Geometry: see drawing. Coordinates: mm, zero at the bounding-box minimum. A direction names the side the tool comes from. Round coordinates to 2 decimals unless told otherwise and drop trailing zeros. Write each loop counter-clockwise with the first axis right and the second up, starting at its lowest first coordinate (ties: lowest second). Pieces come first, ordered by that corner, then holes. Notation, with made-up numbers: (5, 29.5) -> (21, 29.5) arc R24 cw to (21, 47.5) -> close; hole circle Ø3 at (-2.5, -22.5). An arc over 180 degrees is marked (long way). Write item = value, one per line. Start each with the question number.
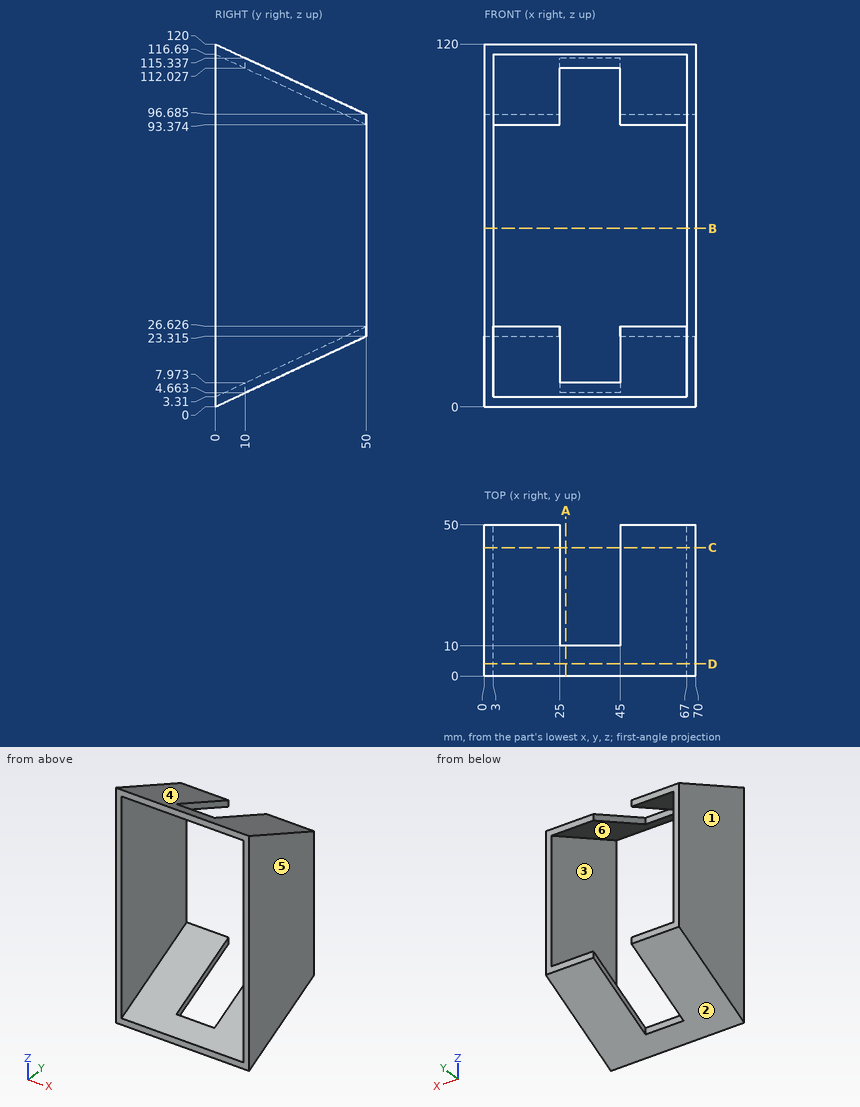
1. Section B-B (z = 59). Output: boundary loops of the cut face in (x, y).
2. Line query: line 1 along X through (y, z) = (7.5, 17); line 2 along Z through (x, y) = (7, 3); line 3 along Z through (x, y) = (5, 29.5) (1 decimal). Output: solid intervals per line, ascending.
3. Mould query, pull axis Z, two halves, no side actions, for the marked faces 1, 2, 3 and 4. Classes: pulls with the +Z half, pulls with the -Z half, needs draft (parallel to the pull), parting line crosses it, or undercut.
4. Reachability of the marked faces 5 and 6 from +Z, -Z, +X, -X, +Y, -Y: full face, straight path, thin tool, end or side. Return the list, or none.
5. Section D-D (y = 4). Output: boundary loops of the cut face in (x, z) (1 decimal), then the cut area to 3 significant figures.
6. Pin query (flat end, axial travel): P1, Ø1.5, axis at x = 62, z = 17.5, coming from the -Y side (1 decimal); P2, Ø5, axis at x = 54, y = 29.5, coming from the -Z side; P3, Ø10, axis at x = 12.5, y = 24.5, coming from the -Z side. Return the tip coordinate at first contact, or that it passes through.
7. Section C-C (y = 42.5). Output: boundary loops of the cut face in (x, z).
8. Section A-A (x = 27). Output: boundary loops of the cut face in (y, z).
Check sheet entries:
q1.outline = (0, 0) -> (3, 0) -> (3, 50) -> (0, 50) -> close; (67, 0) -> (70, 0) -> (70, 50) -> (67, 50) -> close
q2.line_1 = 0 to 3, 67 to 70
q2.line_2 = 1.4 to 4.71, 115.29 to 118.6
q2.line_3 = 13.8 to 17.1, 102.9 to 106.2
q3.face_1 = needs draft
q3.face_2 = pulls with the -Z half
q3.face_3 = undercut
q3.face_4 = pulls with the +Z half
q4.face_5 = +Z, -Z, +X, +Y, -Y
q4.face_6 = -Y
q5.outline = (0, 1.9) -> (70, 1.9) -> (70, 118.1) -> (0, 118.1) -> close; hole (3, 5.2) -> (67, 5.2) -> (67, 114.8) -> (3, 114.8) -> close
q5.area = 1,120 mm2
q6.P1 = 28.8
q6.P2 = 12.59
q6.P3 = 9.09
q7.outline = (0, 19.82) -> (25, 19.82) -> (25, 23.13) -> (3, 23.13) -> (3, 96.87) -> (25, 96.87) -> (25, 100.18) -> (0, 100.18) -> close; (45, 19.82) -> (70, 19.82) -> (70, 100.18) -> (45, 100.18) -> (45, 96.87) -> (67, 96.87) -> (67, 23.13) -> (45, 23.13) -> close
q8.outline = (0, 0) -> (10, 4.66) -> (10, 7.97) -> (0, 3.31) -> close; (0, 116.69) -> (10, 112.03) -> (10, 115.34) -> (0, 120) -> close
